Design review of the part built by this model. Coordinates are the model's own, in mm. Face numbers are marked on the shaded views. A direction names the side the tool comes from. Coordinates: 2 decimals unless noted, no trailing zeros. Write each loop counter-clockwise with the first axis right and the second up, starting at its lowest first coordinate (ties: lowest second). Pieces come first, ordered by that corner, then holes. Notation, with made-up numbers: (28, 29.5) - (63, 29.5) arc R38 cw to (63, 68.5) - close; hole circle Ø6 at (27, -30.5). An arc over 180 degrees is marked (long way). Answer as a JSON object with one key per item and string values.
```python
from build123d import *

# Parameters (mm, degrees)
F1_DEPTH = 6
F3_DEPTH = 0.5
F4_R     = 3
F5_DEPTH = 0.5
F6_DEPTH = 6
F7_R     = 3
F8_R     = 2.99999


# Not quite as in the source:
# - a fillet or chamfer is up to 0.001 mm smaller than in the source, because OpenCascade refuses the exact size


with BuildPart() as f1:
    # F0 (on Front) → F1 (new body)
    with BuildSketch(Plane.XZ):
        with BuildLine():
            Line((-38.9118868113, 40.6996482372), (-38.9118868113, 42.7731432119))
            ThreePointArc((-38.9118868113, 42.7731432119), (-42.3638979782, 40.9564388024), (-44.9301813825, 38.0185849093))
            ThreePointArc((-44.9301813825, 38.0185849093), (-35.7618868113, 21.9496482372), (-26.59359224, 38.0185849093))
            ThreePointArc((-26.59359224, 38.0185849093), (-29.1598756443, 40.9564388024), (-32.6118868113, 42.7731432119))
            Line((-32.6118868113, 42.7731432119), (-32.6118868113, 40.6996482372))
            Line((-32.6118868113, 40.6996482372), (-35.7618868113, 40.6996482372))
            Line((-35.7618868113, 40.6996482372), (-38.9118868113, 40.6996482372))
        make_face()
        with BuildLine():
            ThreePointArc((-35.7618868113, 35.7496482372), (-33.5345004505, 34.827034598), (-32.6118868113, 32.5996482372))
            ThreePointArc((-32.6118868113, 32.5996482372), (-35.7618868113, 29.4496482372), (-38.9118868113, 32.5996482372))
            ThreePointArc((-38.9118868113, 32.5996482372), (-37.989273172, 34.827034598), (-35.7618868113, 35.7496482372))
        make_face(mode=Mode.SUBTRACT)
        with BuildLine():
            ThreePointArc((-44.9301813825, 38.0185849093), (-42.3638979782, 40.9564388024), (-38.9118868113, 42.7731432119))
            Line((-38.9118868113, 42.7731432119), (-38.9118868113, 55.9496482372))
            Line((-38.9118868113, 55.9496482372), (-46.4118868113, 51.5996482372))
            Line((-46.4118868113, 51.5996482372), (-46.4118868113, 42.5996482372))
            ThreePointArc((-46.4118868113, 42.5996482372), (-44.652769306, 40.6384655389), (-44.9301813825, 38.0185849093))
        make_face()
        with BuildLine():
            ThreePointArc((-32.6118868113, 42.7731432119), (-29.1598756443, 40.9564388024), (-26.59359224, 38.0185849093))
            ThreePointArc((-26.59359224, 38.0185849093), (-26.8710043165, 40.6384655389), (-25.1118868113, 42.5996482372))
            Line((-25.1118868113, 42.5996482372), (-25.1118868113, 51.5996482372))
            Line((-25.1118868113, 51.5996482372), (-32.6118868113, 55.9496482372))
            Line((-32.6118868113, 55.9496482372), (-32.6118868113, 42.7731432119))
        make_face()
    extrude(amount=F1_DEPTH)

    # F2 (on face) → F3 (join)
    with BuildSketch(Plane(origin=(-32.6118868113, 0, 0), x_dir=(0, -1, 0), z_dir=(-1, 0, 0))):
        with BuildLine():
            ThreePointArc((3, 54.4897693761), (0.9582631067, 49.3483636635), (6.0587201472, 51.4903441072))
            ThreePointArc((6.0587201472, 51.4903441072), (5.1591771878, 53.6323245508), (3, 54.4897693761))
        make_face()
    extrude(amount=F3_DEPTH)

    # F4 (on face) → F5 (join)
    with BuildSketch(Plane.YZ.offset(-38.9118868113)):
        with Locations((-3.0229054391, 51.2129813433)):
            Circle(F4_R)
    extrude(amount=F5_DEPTH)

    # F0 (on Front) → F6 (join)
    with BuildSketch(Plane.XZ):
        with BuildLine():
            Line((-38.9118868113, 40.6996482372), (-38.9118868113, 42.7731432119))
            ThreePointArc((-38.9118868113, 42.7731432119), (-42.3638979782, 40.9564388024), (-44.9301813825, 38.0185849093))
            ThreePointArc((-44.9301813825, 38.0185849093), (-35.7618868113, 21.9496482372), (-26.59359224, 38.0185849093))
            ThreePointArc((-26.59359224, 38.0185849093), (-29.1598756443, 40.9564388024), (-32.6118868113, 42.7731432119))
            Line((-32.6118868113, 42.7731432119), (-32.6118868113, 40.6996482372))
            Line((-32.6118868113, 40.6996482372), (-35.7618868113, 40.6996482372))
            Line((-35.7618868113, 40.6996482372), (-38.9118868113, 40.6996482372))
        make_face()
        with BuildLine():
            ThreePointArc((-35.7618868113, 35.7496482372), (-33.5345004505, 34.827034598), (-32.6118868113, 32.5996482372))
            ThreePointArc((-32.6118868113, 32.5996482372), (-35.7618868113, 29.4496482372), (-38.9118868113, 32.5996482372))
            ThreePointArc((-38.9118868113, 32.5996482372), (-37.989273172, 34.827034598), (-35.7618868113, 35.7496482372))
        make_face(mode=Mode.SUBTRACT)
        with BuildLine():
            ThreePointArc((-44.9301813825, 38.0185849093), (-42.3638979782, 40.9564388024), (-38.9118868113, 42.7731432119))
            Line((-38.9118868113, 42.7731432119), (-38.9118868113, 55.9496482372))
            Line((-38.9118868113, 55.9496482372), (-46.4118868113, 51.5996482372))
            Line((-46.4118868113, 51.5996482372), (-46.4118868113, 42.5996482372))
            ThreePointArc((-46.4118868113, 42.5996482372), (-44.652769306, 40.6384655389), (-44.9301813825, 38.0185849093))
        make_face()
        with BuildLine():
            ThreePointArc((-32.6118868113, 42.7731432119), (-29.1598756443, 40.9564388024), (-26.59359224, 38.0185849093))
            ThreePointArc((-26.59359224, 38.0185849093), (-26.8710043165, 40.6384655389), (-25.1118868113, 42.5996482372))
            Line((-25.1118868113, 42.5996482372), (-25.1118868113, 51.5996482372))
            Line((-25.1118868113, 51.5996482372), (-32.6118868113, 55.9496482372))
            Line((-32.6118868113, 55.9496482372), (-32.6118868113, 42.7731432119))
        make_face()
    extrude(amount=F6_DEPTH)

    # F7
    f7_edges = [f1.edges().sort_by_distance(p)[0] for p in [
        (-35.761887, -6, 40.699648),
    ]]
    fillet(f7_edges, radius=F7_R)

    # F8 (radius 3 in the source; OpenCascade refuses exactly that, so slightly less here)
    f8_edges = [f1.edges().sort_by_distance(p)[0] for p in [
        (-35.761887, 0, 40.699648),
    ]]
    fillet(f8_edges, radius=F8_R)


solid = f1.part
```
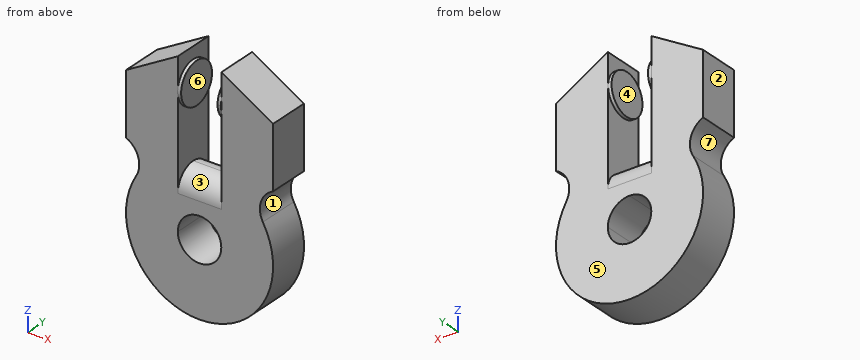
(1) The part is to be moulded in two halves that separate along X. For the marked faces 5, 6 and 7, say which applies: pulls with the +X half, pulls with the -X half, needs draft (parallel to the pull), parting line crosses it, or undercut.
Solved:
{"face 5": "needs draft", "face 6": "undercut", "face 7": "pulls with the -X half"}
(2) Tool access review of the marked faces 1, 2, 3 and 4: name each direction out of +Z, -Z, +X, -X, +Y, -Y from which nothing blocks a thin tool from reaching the whole face with its end or side.
Solved:
{"face 1": "+X, +Y, -Y", "face 2": "+Z, -Z, -X, +Y, -Y", "face 3": "-Y", "face 4": "+Z, +Y, -Y"}
(3) Take a section at A-A, the plane z = 46. Write out the cut boundary in (x, y), and give its area (3 significant figures).
Solved:
{"outline": "(-46.41, -6) - (-38.91, -6) - (-38.91, 0) - (-46.41, 0) - close; (-32.61, -6) - (-25.11, -6) - (-25.11, 0) - (-32.61, 0) - close", "area": "90.0 mm^2"}
(4) Take a section at B-B, the plane y = -4. Write out the cut boundary in (x, z), and give its area (3 significant figures).
Solved:
{"outline": "(-46.41, 42.6) arc R3.24 cw to (-44.93, 38.02) arc R10.65 ccw (long way) to (-26.59, 38.02) arc R3.24 cw to (-25.11, 42.6) - (-25.11, 51.6) - (-32.61, 55.95) - (-32.61, 54.34) - (-33.11, 54.34) - (-33.11, 48.64) - (-32.61, 48.64) - (-32.61, 40.53) - (-38.91, 40.53) - (-38.91, 48.38) - (-38.41, 48.38) - (-38.41, 54.05) - (-38.91, 54.05) - (-38.91, 55.95) - (-46.41, 51.6) - close; hole circle Ø6.3 at (-35.76, 32.6)", "area": "501 mm^2"}
(5) For pin 1 (6.5 mm diameter, centred on x = -36.5, z = 37.5, fed in from -Y); pin 2 (2 mm diameter, centred on x = -41.5, y = -4.5, fed in from +Z); pin 3 (1.8 mm diameter, centred on y = -3.5, z = 42.5, fed in from -X); pin 4 (2 mm diameter, centred on x = -41.5, y = -1, fed in from -Z), all flat-tipped, find the tip position at first contact; note any pin that passes through.
Solved:
{"pin 1": "stops at y = -6", "pin 2": "stops at z = 55.03", "pin 3": "stops at x = -46.41", "pin 4": "stops at z = 23.06"}
(6) To check wall thickness, follow line 1 (X direction, y = -0.75, z = 49); line 2 (Z direction, x = -38, y = -0.25); line 3 (X direction, y = -3.75, z = 34). State the ranges of each line that lie inside material, in increasing order. Write a range as from..to.
Solved:
{"line 1": "x = -46.41..-38.91, -32.61..-25.11", "line 2": "z = 22.19..30.38, 34.82..38.9", "line 3": "x = -46.32..-38.58, -32.94..-25.2"}
(7) Take a section at D-D, the plane z = 34.5. Write out the cut boundary in (x, y).
Solved:
{"outline": "(-46.24, -6) - (-38.27, -6) - (-38.27, 0) - (-46.24, 0) - close; (-33.25, -6) - (-25.28, -6) - (-25.28, 0) - (-33.25, 0) - close"}
